Geometry check sheet. Reference: the model listing, model coordinates, mm. Face numbers are marked on the shaded views. A direction names the side the tool comes from. Round coordinates to 2 decimals unless told otherwise and drop trailing zeros. Write each loop counter-clockwise with the first axis right and the second up, starting at its lowest first coordinate (ties: lowest second). Pieces come first, ordered by that corner, then holes. Notation, with made-up numbers: M 26.5,54 L 42.5,54 A15 cw 42.5,79 Z; hole C 1,47.25 d6. An arc over 180 degrees is marked long. Answer as CSV lines item,"result". Start each with the question number.
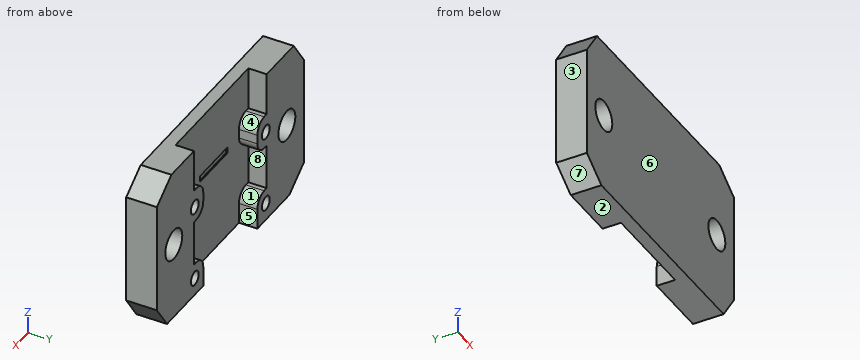
```python
from build123d import *
from OCP.BRepFilletAPI import BRepFilletAPI_MakeChamfer

# Parameters (mm, degrees)
SKETCH2_W           = 25.4
SKETCH2_H           = 25.4
BOSS_EXTRUDE6_DEPTH = 5
BOSS_EXTRUDE7_DEPTH = 5
FILLET1_R           = 5
SKETCH5_R           = 1
CUT_EXTRUDE1_DEPTH  = 5
SKETCH6_W           = 28.098270468
SKETCH6_H           = 9.80175879
CUT_EXTRUDE2_DEPTH  = 49.905214446
SKETCH7_W           = 43.4
SKETCH7_H           = 25.4
SKETCH7_R           = 2.5
BOSS_EXTRUDE8_DEPTH = 5
SKETCH8_R           = 2.5
CUT_EXTRUDE3_DEPTH  = 10
SKETCH9_R           = 1.15
CUT_EXTRUDE4_DEPTH  = 3
FILLET2_R           = 2
CHAMFER1_SIZE       = 3
CHAMFER1_SIZE2      = 4.28444402
SKETCH10_W          = 8.049726934
SKETCH10_H          = 1.005360961
CUT_EXTRUDE5_DEPTH  = 0.2


with BuildPart() as part:
    # Sketch2 → Boss-Extrude6 (new body)
    with BuildSketch(Plane(origin=(0, 0, 0), x_dir=(1, 0, 0), z_dir=(0, 1, 0))):
        with Locations((12.7, 12.7)):
            Rectangle(SKETCH2_W, SKETCH2_H)
    extrude(amount=BOSS_EXTRUDE6_DEPTH)

    # Sketch4 → Boss-Extrude7 (add)
    with BuildSketch(Plane.XZ):
        with BuildLine():
            Line((25.4, 0), (25.4, -9.7))
            ThreePointArc((25.4, -9.7), (34.4, -12.7), (25.4, -15.7))
            Line((25.4, -15.7), (25.4, -25.4))
            Line((25.4, -25.4), (15.7, -25.4))
            ThreePointArc((15.7, -25.4), (12.7, -34.4), (9.7, -25.4))
            Line((9.7, -25.4), (0, -25.4))
            Line((0, -25.4), (0, -15.7))
            ThreePointArc((0, -15.7), (-9, -12.7), (0, -9.7))
            Line((0, -9.7), (0, 0))
            Line((0, 0), (9.7, 0))
            Line((9.7, 0), (15.7, 0))
            Line((15.7, 0), (25.4, 0))
        make_face()
    extrude(amount=-BOSS_EXTRUDE7_DEPTH)

    # Fillet1
    fillet1_edges = [part.edges().sort_by_distance(p)[0] for p in [
        (25.4, 2.5, -9.7),
        (25.4, 2.5, -15.7),
        (15.7, 2.5, -25.4),
        (9.7, 2.5, -25.4),
        (0, 2.5, -15.7),
        (0, 2.5, -9.7),
    ]]
    fillet(fillet1_edges, radius=FILLET1_R)

    # Sketch5 → Cut-Extrude1 (cut)
    with BuildSketch(Plane(origin=(0, 5, 0), x_dir=(1, 0, 0), z_dir=(0, 1, 0))):
        with Locations(Location((-4, 12.7, 0), (0, 0, 270))):
            Circle(SKETCH5_R)
        with Locations(Location((12.7, 29.4, 0), (0, 0, 270))):
            Circle(SKETCH5_R)
        with Locations(Location((29.4, 12.7, 0), (0, 0, 270))):
            Circle(SKETCH5_R)
    extrude(amount=-CUT_EXTRUDE1_DEPTH, mode=Mode.SUBTRACT)

    # Sketch6 → Cut-Extrude2 (cut, through all)
    with BuildSketch(Plane(origin=(0, 5, 0), x_dir=(1, 0, 0), z_dir=(0, 1, 0))):
        with Locations((14.049135234, 30.300879395)):
            Rectangle(SKETCH6_W, SKETCH6_H)
    extrude(amount=-CUT_EXTRUDE2_DEPTH, mode=Mode.SUBTRACT)

    # Sketch7 → Boss-Extrude8 (add)
    with BuildSketch(Plane(origin=(0, 5, 0), x_dir=(1, 0, 0), z_dir=(0, 1, 0))):
        with Locations((12.7, 12.7)):
            Rectangle(SKETCH7_W, SKETCH7_H)
        with Locations((-4, 12.7)):
            Circle(SKETCH7_R, mode=Mode.SUBTRACT)
        with Locations((29.4, 12.7)):
            Circle(SKETCH7_R, mode=Mode.SUBTRACT)
    extrude(amount=-BOSS_EXTRUDE8_DEPTH)

    # Sketch8 → Cut-Extrude3 (cut)
    with BuildSketch(Plane(origin=(0, 5, 0), x_dir=(1, 0, 0), z_dir=(0, 1, 0))):
        with Locations(Location((-4, 12.7, 0), (0, 0, 270))):
            Circle(SKETCH8_R)
        with Locations(Location((29.4, 12.7, 0), (0, 0, 270))):
            Circle(SKETCH8_R)
    extrude(amount=-CUT_EXTRUDE3_DEPTH, mode=Mode.SUBTRACT)

    # Sketch9 → Cut-Extrude4 (cut)
    with BuildSketch(Plane(origin=(0, 5, 0), x_dir=(1, 0, 0), z_dir=(0, 1, 0))):
        with Locations(Location((2.2, 10, 0), (0, 0, 270))):
            Circle(SKETCH9_R)
        with Locations(Location((2.2, 22.5, 0), (0, 0, 270))):
            Circle(SKETCH9_R)
        with Locations(Location((23.2, 22.5, 0), (0, 0, 270))):
            Circle(SKETCH9_R)
        with Locations(Location((23.2, 10, 0), (0, 0, 270))):
            Circle(SKETCH9_R)
        Polygon((23.45, 12.5), (23.45, 20), (20.7, 20), (20.7, 25.4), (4.7, 25.4), (4.7, 20), (1.95, 20), (1.95, 12.5), (4.7, 12.5), (4.7, 7), (1.95, 7), (1.95, 0), (23.45, 0), (23.45, 7), (20.7, 7), (20.7, 12.5), align=None)
    extrude(amount=-CUT_EXTRUDE4_DEPTH, mode=Mode.SUBTRACT)

    # Fillet2
    fillet2_edges = [part.edges().sort_by_distance(p)[0] for p in [
        (20.7, 3.5, -12.5),
        (20.7, 3.5, -7),
        (4.7, 3.5, -7),
        (4.7, 3.5, -12.5),
        (4.7, 3.5, -20),
        (20.7, 3.5, -20),
    ]]
    fillet(fillet2_edges, radius=FILLET2_R)

    # Chamfer1: one chamfer whose edges measure the first distance from different faces: ONE call of the kernel's chamfer builder (chamfer() names one face for all edges)
    chamfer1_edges_1 = [part.edges().sort_by_distance(p)[0] for p in [
        (34.4, 2.5, 0),
    ]]
    chamfer1_side_1 = [part.faces().sort_by_distance(p)[0] for p in [
        (34.4, 2.5, -12.7),
    ]]
    chamfer1_edges_2 = [part.edges().sort_by_distance(p)[0] for p in [
        (-9, 2.5, 0),
    ]]
    chamfer1_side_2 = [part.faces().sort_by_distance(p)[0] for p in [
        (-8.56312931, 2.5, 0),
    ]]
    chamfer1_edges_3 = [part.edges().sort_by_distance(p)[0] for p in [
        (34.4, 2.5, -25.4),
    ]]
    chamfer1_side_3 = [part.faces().sort_by_distance(p)[0] for p in [
        (33.96312931, 2.5, -25.4),
    ]]
    chamfer1_edges_4 = [part.edges().sort_by_distance(p)[0] for p in [
        (-9, 2.5, -25.4),
    ]]
    chamfer1_side_4 = [part.faces().sort_by_distance(p)[0] for p in [
        (-9, 2.5, -12.7),
    ]]
    chamfer1 = BRepFilletAPI_MakeChamfer(part.part.solid().wrapped)
    for e in chamfer1_edges_1:
        chamfer1.Add(CHAMFER1_SIZE, CHAMFER1_SIZE2, e.wrapped, chamfer1_side_1[0].wrapped)  # the first distance lies on this face
    for e in chamfer1_edges_2:
        chamfer1.Add(CHAMFER1_SIZE, CHAMFER1_SIZE2, e.wrapped, chamfer1_side_2[0].wrapped)  # the first distance lies on this face
    for e in chamfer1_edges_3:
        chamfer1.Add(CHAMFER1_SIZE, CHAMFER1_SIZE2, e.wrapped, chamfer1_side_3[0].wrapped)  # the first distance lies on this face
    for e in chamfer1_edges_4:
        chamfer1.Add(CHAMFER1_SIZE, CHAMFER1_SIZE2, e.wrapped, chamfer1_side_4[0].wrapped)  # the first distance lies on this face
    add(Compound.cast(chamfer1.Shape()), mode=Mode.REPLACE)

    # Sketch10 → Cut-Extrude5 (cut)
    with BuildSketch(Plane(origin=(0, 2, 0), x_dir=(1, 0, 0), z_dir=(0, 1, 0))):
        with Locations((12.181188926, 10.502680481)):
            Rectangle(SKETCH10_W, SKETCH10_H)
    extrude(amount=-CUT_EXTRUDE5_DEPTH, mode=Mode.SUBTRACT)


solid = part.part
```
1) Section check D-D, the plane y = 4.2. Give the number of separate pieces and of enclosed holes in the cut face, plus the area to 3 significant figures.
2) Section check B-B, the plane y = 0.55. Record the cut outline in (x, z), plus the area to 3 significant figures.
3) Access from +Z, -Z, +X, -X, +Y, -Y to the whole of each face (thin tool, end or side, straight path). Record for the marked faces 1, 2, 3, 4 and 5.
4) Scan lines: line 1 (X direction, y = 3.55, z = -12.7); line 2 (X direction, y = 1.4, z = -12.7); line 3 (X direction, y = 3.95, z = -22.5). Record each from-to range of solid material in increasing order. Write a range as from..to.
5) Mould release check, pull along Z, two halves, no side actions. Record for the marked faces 6, 7 and 8: released by +Z, released by -Z, zero draft, split by the parting line, or undercut.
6) Section check A-A, the plane x = -4. Record the cut outline in (y, z), plus the area to 3 significant figures.
7) Go/stop test with flat-tipped pins: pin 1 (3 mm diameter, centred on x = 2.2, z = -10, fed in from -Y); pin 2 (0.8 mm diameter, centred on x = 23, y = 4, fed in from +Z); pin 3 (0.7 mm diameter, centred on x = 23.5, z = -22, fed in from +Y); pin 4 (0.9 mm diameter, centred on y = 4, z = -23.5, fed in from +X). Record where each tip stops, or that it passes through.
8) Section check C-C, the plane x = 15.5. Record the cut outline in (y, z), plus the area to 3 significant figures.
Results:
1,separate pieces,"2"
1,enclosed holes,"6"
1,area,"529 mm^2"
2,outline,"M -9,-22.4 L -4.72,-25.4 L 31.4,-25.4 L 34.4,-21.12 L 34.4,-3 L 30.12,0 L -6,0 L -9,-4.28 Z; hole C -4,-12.7 d5; hole C 29.4,-12.7 d5"
2,area,"1,040 mm^2"
3,face 1,"+Y"
3,face 2,"-Z, +X, -X, +Y, -Y"
3,face 3,"+Z, -Z, -X, +Y, -Y"
3,face 4,"+Z, +Y"
3,face 5,"+Z, -Z, +Y"
4,line 1,"x = -9..-6.5, -1.5..1.95, 23.45..26.9, 31.9..34.4"
4,line 2,"x = -9..-6.5, -1.5..26.9, 31.9..34.4"
4,line 3,"x = -8.86..1.05, 3.35..4.7, 20.7..22.05, 24.35..33.43"
5,face 6,"zero draft"
5,face 7,"released by -Z"
5,face 8,"undercut"
6,outline,"M 0,-25.4 L 5,-25.4 L 5,-15.2 L 0,-15.2 Z; M 0,-10.2 L 5,-10.2 L 5,0 L 0,0 Z"
6,area,"102 mm^2"
7,pin 1,"stops at y = 0"
7,pin 2,"stops at z = -7"
7,pin 3,"stops at y = 2"
7,pin 4,"stops at x = 33.05"
8,outline,"M 0,-25.4 L 2,-25.4 L 2,-11.01 L 1.8,-11.01 L 1.8,-10 L 2,-10 L 2,0 L 0,0 Z"
8,area,"50.6 mm^2"
